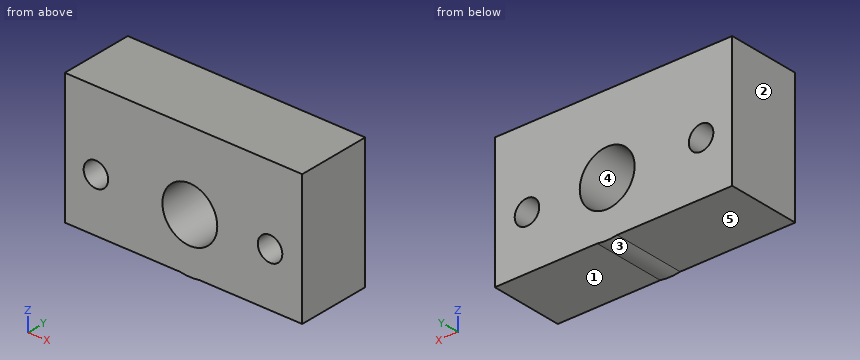
```python
from build123d import *

# Parameters (mm, degrees)
F0_R     = 14.1997272149
F0_R_2   = 6.35
F2_DEPTH = 12.7
F3_DEPTH = 25.4


# Not quite as in the source:
# - the program builds the solid bodies; features that only make, move or delete a surface that nothing else refers to are left out


with BuildPart() as f2:
    # F0 (on Front) → F2 (new body)
    with BuildSketch(Plane.XZ):
        with BuildLine():
            ThreePointArc((5.1667592351, -27.8533101082), (21.7815136707, -18.1126460571), (28.3284712785, 0))
            ThreePointArc((28.3284712785, 0), (-18.1126460571, 21.7815136707), (-5.1667592351, -27.8533101082))
            Line((-5.1667592351, -27.8533101082), (5.1667592351, -27.8533101082))
        make_face()
        Circle(F0_R, mode=Mode.SUBTRACT)
        with BuildLine():
            ThreePointArc((-5.1667592351, -27.8533101082), (-18.1126460571, 21.7815136707), (28.3284712785, 0))
            ThreePointArc((28.3284712785, 0), (21.7815136707, -18.1126460571), (5.1667592351, -27.8533101082))
            Line((5.1667592351, -27.8533101082), (58.1642687321, -27.8533101082))
            Line((58.1642687321, -27.8533101082), (58.1642687321, 40.1415377855))
            Line((58.1642687321, 40.1415377855), (-64.7179856896, 40.1415377855))
            Line((-64.7179856896, 40.1415377855), (-64.7179856896, -27.8533101082))
            Line((-64.7179856896, -27.8533101082), (-5.1667592351, -27.8533101082))
        make_face()
        with Locations((-48.6067570746, 0)):
            Circle(F0_R_2, mode=Mode.SUBTRACT)
        with Locations((41.5068976581, 0)):
            Circle(F0_R_2, mode=Mode.SUBTRACT)
        with BuildLine():
            Line((5.1667592351, -27.8533101082), (-5.1667592351, -27.8533101082))
            ThreePointArc((-5.1667592351, -27.8533101082), (0, -28.3284712785), (5.1667592351, -27.8533101082))
        make_face()
    extrude(amount=F2_DEPTH)

    # F3 (add): a face of the model
    f3_faces = [f2.faces().sort_by_distance(p)[0] for p in [
        (56.7575636957, -12.7, 6.1441138387),
    ]]
    extrude(f3_faces, amount=F3_DEPTH)


solid = f2.part
```
Could you check a few things on this model? Use its own coordinates, in mm. Face numbers are marked on the shaded views. A direction names the side the tool comes from. Give positions to 0.01 mm unless a question says otherwise; leave off trailing zeros. Loops run counter-clockwise (first coordinate to the right, second up) from the corner with the lowest first, then second, coordinate; pieces in that order, holes last. Notation, with made-up numbers: (3, 21.25) - (60, 21.25) arc R28 ccw to (60, 41.25) - close; hole circle Ø4 at (80, 44). An arc over 180 degrees is marked (long way). Answer in a Markdown table with one row per item. Add a question column.
Q1. For pin 1 (16.5 mm diameter, centred on x = -48.61, z = 0, fed in from -Y); pin 2 (10 mm diameter, centred on x = -46, y = -15, fed in from -Z), each with a flat end and sliding along its axis, tell me the tip position at first contact or that it passes through.
Q2. We'd pull the mould along X, two halves only. Please class the marked faces 3, 4 and 5: +X half, -X half, draft (parallel to the pull), parting line (faces both ways), or undercut.
Q3. Which directions (+Z, -Z, +X, -X, +Y, -Y) give clear straight access to the entire face, cutting with the end or side of a thin tool? Please do the marked faces 1 and 2.
Q4. If we section it at D-D (x = 12.5): List the corners of the cut face in (y, z) for me, plus the area to 3 significant figures.
Q5. If we section it at A-A (z = 0): List the corners of the cut face in (x, y) for me.
Q6. If we section it at B-B (x = 0): List the corners of the cut face in (y, z) for me, plus the area to 3 significant figures.
Q7. If we section it at C-C (y = -2.5): List the corners of the cut face in (x, z) for me.
Q8. Please list where these lines run through material, in increasing order: L1, parallel to Z at x = 0, y = -14; L2, parallel to X at y = -18, z = 2; L3, parallel to X at y = -24, z = 5. Write a range as from..to.
The answers:
| question | item | result |
|---|---|---|
| 1 | pin 1 | stops at y = -38.1 |
| 1 | pin 2 | stops at z = -27.85 |
| 2 | face 3 | parting line |
| 2 | face 4 | undercut |
| 2 | face 5 | draft |
| 3 | face 1 | -Z, +X, +Y, -Y |
| 3 | face 2 | +Z, -Z, -X, +Y, -Y |
| 4 | outline | (-38.1, -27.85) - (0, -27.85) - (0, -6.74) - (-38.1, -6.74) - close; (-38.1, 6.74) - (0, 6.74) - (0, 40.14) - (-38.1, 40.14) - close |
| 4 | area | 2,080 mm^2 |
| 5 | outline | (-64.72, -38.1) - (-54.96, -38.1) - (-54.96, 0) - (-64.72, 0) - close; (-42.26, -38.1) - (-14.2, -38.1) - (-14.2, 0) - (-42.26, 0) - close; (14.2, -38.1) - (35.16, -38.1) - (35.16, 0) - (14.2, 0) - close; (47.86, -38.1) - (58.16, -38.1) - (58.16, 0) - (47.86, 0) - close |
| 6 | outline | (-38.1, -28.33) - (0, -28.33) - (0, -14.2) - (-38.1, -14.2) - close; (-38.1, 14.2) - (0, 14.2) - (0, 40.14) - (-38.1, 40.14) - close |
| 6 | area | 1,530 mm^2 |
| 7 | outline | (-64.72, -27.85) - (-5.17, -27.85) arc R28.33 ccw to (5.17, -27.85) - (58.16, -27.85) - (58.16, 40.14) - (-64.72, 40.14) - close; hole circle Ø12.7 at (-48.61, 0); hole circle Ø28.4 at (0, 0); hole circle Ø12.7 at (41.51, 0) |
| 8 | L1 | z = -28.33..-14.2, 14.2..40.14 |
| 8 | L2 | x = -64.72..-54.63, -42.58..-14.06, 14.06..35.48, 47.53..58.16 |
| 8 | L3 | x = -64.72..-52.52, -44.69..-13.29, 13.29..37.59, 45.42..58.16 |
